Source: three-view drawing plus pictorial views. Frame: mm from the lowest corner of the part. Give positions to 0.01 mm unless a question says otherwise; leave off trailing zeros. Order: outer loops, then holes, each group sorted by start corner. A loop starts at its lowest first (then second) coordinate and runs counter-clockwise, first axis right, second up. Notation, with made-up numbers: (-5.5, -30) -> (31.5, -30) arc R18 ccw to (31.5, -11) -> close; hole circle Ø7 at (-26.5, 33). An arc over 180 degrees is marked (long way). Write item = value, one per line.
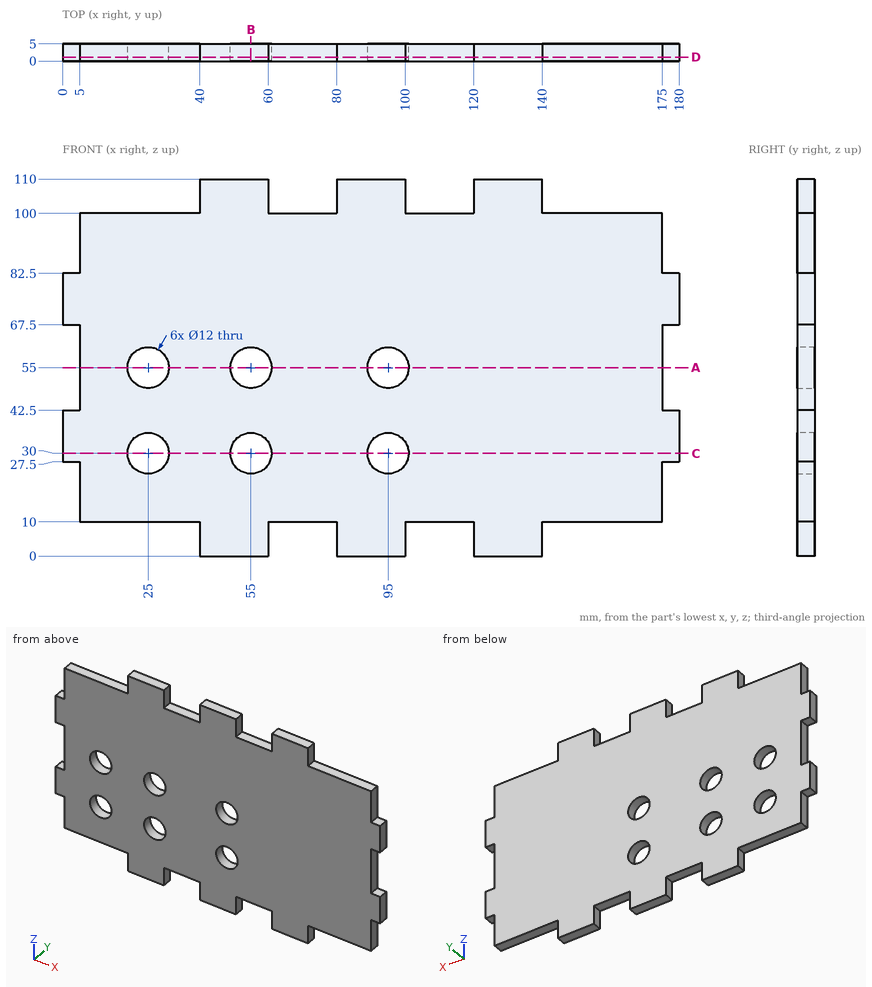
1) First-contact query: P1, Ø1.5, axis at y = 2.5, z = 105, coming from the +X side; P2, Ø2.5, axis at y = 2.5, z = 56.5, coming from the -X side; P3, Ø2.5, axis at x = 69.5, y = 3.5, coming from the -Z side; P4, Ø11, axis at x = 95, z = 30, coming from the +Y side. Flat tips, straight axial feed; report the tip coordinate or a pass-through.
Check sheet entries:
P1 = 140
P2 = 5
P3 = 10
P4 = through
2) Section query B-B (x = 55). Output: boundary loops of the cut face in (y, z).
Check sheet entries:
outline = (0, 0) -> (5, 0) -> (5, 24) -> (0, 24) -> close; (0, 36) -> (5, 36) -> (5, 49) -> (0, 49) -> close; (0, 61) -> (5, 61) -> (5, 110) -> (0, 110) -> close
3) Section query A-A (z = 55). Output: boundary loops of the cut face in (x, y), plus the area to 3 significant figures.
Check sheet entries:
outline = (5, 0) -> (19, 0) -> (19, 5) -> (5, 5) -> close; (31, 0) -> (49, 0) -> (49, 5) -> (31, 5) -> close; (61, 0) -> (89, 0) -> (89, 5) -> (61, 5) -> close; (101, 0) -> (175, 0) -> (175, 5) -> (101, 5) -> close
area = 670 mm²
4) Section query C-C (z = 30). Output: boundary loops of the cut face in (x, y).
Check sheet entries:
outline = (0, 0) -> (19, 0) -> (19, 5) -> (0, 5) -> close; (31, 0) -> (49, 0) -> (49, 5) -> (31, 5) -> close; (61, 0) -> (89, 0) -> (89, 5) -> (61, 5) -> close; (101, 0) -> (180, 0) -> (180, 5) -> (101, 5) -> close
5) Section query D-D (y = 1.2). Count the separate pieces of the cut face and the enclosed holes in it, plus the area to 3 significant figures.
Check sheet entries:
separate_pieces = 1
enclosed_holes = 6
area = 16,100 mm²
6) Line query: line 1 (Z direction, x = 95.5, y = 4.1); line 2 (X direction, y = 2.7, z = 55); line 3 (X direction, y = 2.85, z = 30). Output: solid intervals per line, ascending. Write a range as from..to.
Check sheet entries:
line_1 = 0..24.02, 35.98..49.02, 60.98..110
line_2 = 5..19, 31..49, 61..89, 101..175
line_3 = 0..19, 31..49, 61..89, 101..180
